Study the drawing (mm; zero at the part's minimum x, y, z) and answer. Coordinates: 2 decimals unless noted, no trailing zeros. Loops run counter-clockwise (first coordinate to the right, second up) from the corner with the lowest first, then second, coordinate; pieces in that order, holes last. Notation, with made-up numbers: (59, 68) -> (104, 68) arc R23 cw to (104, 88) -> close; hole circle Ø1 at (-11.75, 87.5). An arc over 180 degrees is marked (long way). One line per question, with ' | ' between items.
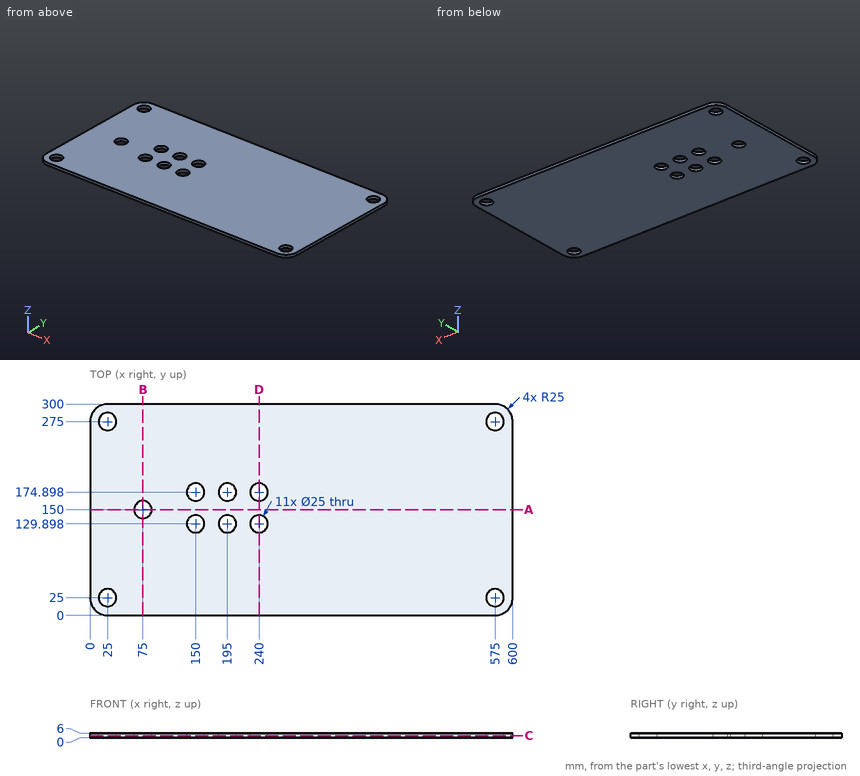
1) Find section D-D (x = 240). Write down the section's boundary in (y, z).
Check values:
outline: (0, 0) -> (117.4, 0) -> (117.4, 6) -> (0, 6) -> close; (142.4, 0) -> (162.4, 0) -> (162.4, 6) -> (142.4, 6) -> close; (187.4, 0) -> (300, 0) -> (300, 6) -> (187.4, 6) -> close
2) Find section A-A (y = 150). Write down the section's boundary in (x, z).
Check values:
outline: (0, 0) -> (62.5, 0) -> (62.5, 6) -> (0, 6) -> close; (87.5, 0) -> (600, 0) -> (600, 6) -> (87.5, 6) -> close
3) Find section B-B (x = 75). Write down the section's boundary in (y, z).
Check values:
outline: (0, 0) -> (137.5, 0) -> (137.5, 6) -> (0, 6) -> close; (162.5, 0) -> (300, 0) -> (300, 6) -> (162.5, 6) -> close
4) Find section C-C (z = 2.7). State how many separate pieces and enclosed holes the cut face has, plus the area to 3 significant figures.
Check values:
separate pieces: 1 | enclosed holes: 11 | area: 174,000 mm^2
5) Find the intervals of material crossed by line 1 along Y through (x, z) = (195, 4.55); line 2 along Y through (x, z) = (575, 2.1); line 3 along X through (y, z) = (150, 3.05), in increasing order.
Check values:
line 1: y = 0 to 117.4, 142.4 to 162.4, 187.4 to 300 | line 2: y = 0 to 12.5, 37.5 to 262.5, 287.5 to 300 | line 3: x = 0 to 62.5, 87.5 to 600
